The listing builds one solid part. Answer for the finished solid, in the listing's coordinates (mm). A direction names the side the tool comes from. Coordinates: 2 decimals unless noted, no trailing zeros. Write each loop counter-clockwise with the first axis right and the second up, starting at its lowest first coordinate (ties: lowest second). Pieces come first, ordered by that corner, then holes.
from build123d import *

# Parameters (mm, degrees)
SKIZZE1_R                       = 1.25
AUFSATZ_LINEAR_AUSTRAGEN1_DEPTH = 2
SKIZZE2_W                       = 150
SKIZZE2_H                       = 52
AUFSATZ_LINEAR_AUSTRAGEN2_DEPTH = 2
SKIZZE3_W                       = 30
SKIZZE3_H                       = 20
SCHNITT_LINEAR_AUSTRAGEN1_DEPTH = 2
SKIZZE5_R                       = 1.25
SCHNITT_LINEAR_AUSTRAGEN2_DEPTH = 2


with BuildPart() as part:
    # Skizze1 → Aufsatz-Linear austragen1 (new body)
    # profile 1 of 2: a face of its own
    with BuildSketch(Plane.XY):
        with BuildLine():
            Line((148, 39.858571571), (148, 12.141428429))
            ThreePointArc((148, 12.141428429), (147.219544457, 8.268445082), (145, 5))
            ThreePointArc((145, 5), (141.731554918, 2.780455543), (137.858571571, 2))
            Line((137.858571571, 2), (12.141428429, 2))
            ThreePointArc((12.141428429, 2), (8.268445082, 2.780455543), (5, 5))
            ThreePointArc((5, 5), (2.780455543, 8.268445082), (2, 12.141428429))
            Line((2, 12.141428429), (2, 39.858571571))
            ThreePointArc((2, 39.858571571), (2.780455543, 43.731554918), (5, 47))
            Line((5, 47), (5, 52))
            Line((5, 52), (145, 52))
            Line((145, 52), (145, 47))
            ThreePointArc((145, 47), (147.219544457, 43.731554918), (148, 39.858571571))
        make_face()
    # profile 2 of 2: a face of its own
    with BuildSketch(Plane.XY):
        with BuildLine():
            ThreePointArc((148, 39.858571571), (147.219544457, 43.731554918), (145, 47))
            Line((145, 47), (145, 52))
            Line((145, 52), (150, 52))
            Line((150, 52), (150, 0))
            Line((150, 0), (0, 0))
            Line((0, 0), (0, 52))
            Line((0, 52), (5, 52))
            Line((5, 52), (5, 47))
            ThreePointArc((5, 47), (2.780455543, 43.731554918), (2, 39.858571571))
            Line((2, 39.858571571), (2, 12.141428429))
            ThreePointArc((2, 12.141428429), (2.780455543, 8.268445082), (5, 5))
            ThreePointArc((5, 5), (8.268445082, 2.780455543), (12.141428429, 2))
            Line((12.141428429, 2), (137.858571571, 2))
            ThreePointArc((137.858571571, 2), (141.731554918, 2.780455543), (145, 5))
            ThreePointArc((145, 5), (147.219544457, 8.268445082), (148, 12.141428429))
            Line((148, 12.141428429), (148, 39.858571571))
        make_face()
        with Locations((2.5, 49.5)):
            Circle(SKIZZE1_R, mode=Mode.SUBTRACT)
        with Locations((2.5, 2.5)):
            Circle(SKIZZE1_R, mode=Mode.SUBTRACT)
        with Locations((147.5, 49.5)):
            Circle(SKIZZE1_R, mode=Mode.SUBTRACT)
        with Locations((147.5, 2.5)):
            Circle(SKIZZE1_R, mode=Mode.SUBTRACT)
    extrude(amount=AUFSATZ_LINEAR_AUSTRAGEN1_DEPTH)

    # Skizze2 → Aufsatz-Linear austragen2 (add)
    with BuildSketch(Plane(origin=(0, 52, 0), x_dir=(1, 0, 0), z_dir=(0, 1, 0))):
        with Locations((75, 24)):
            Rectangle(SKIZZE2_W, SKIZZE2_H)
    extrude(amount=AUFSATZ_LINEAR_AUSTRAGEN2_DEPTH)

    # Skizze3 → Schnitt-Linear austragen1 (cut)
    with BuildSketch(Plane.XZ.offset(-52)):
        with Locations((115, -40)):
            Rectangle(SKIZZE3_W, SKIZZE3_H)
    extrude(amount=-SCHNITT_LINEAR_AUSTRAGEN1_DEPTH, mode=Mode.SUBTRACT)

    # Skizze5 → Schnitt-Linear austragen2 (cut)
    with BuildSketch(Plane(origin=(0, 54, 0), x_dir=(1, 0, 0), z_dir=(0, 1, 0))):
        with Locations(Location((147.5, 47.5, 0), (0, 0, 270))):
            Circle(SKIZZE5_R)
        with Locations(Location((2.5, 47.5, 0), (0, 0, 270))):
            Circle(SKIZZE5_R)
    extrude(amount=-SCHNITT_LINEAR_AUSTRAGEN2_DEPTH, mode=Mode.SUBTRACT)


solid = part.part
1. Flat-ended cylindrical pins translate along their axes: P1, Ø2, axis at x = 147.5, y = 2.5, coming from the -Z side; P2, Ø15.5, axis at x = 108.5, y = 20.5, coming from the -Z side; P3, Ø3, axis at x = 147.5, z = -47.5, coming from the -Y side; P4, Ø1.6, axis at x = 116.5, y = 53.5, coming from the -Z side. Find the tip coordinate at first contact, or state that the pin passes through.
Results found:
P1: passes through
P2: stops at z = 0
P3: stops at y = 52
P4: stops at z = -30
2. A tool of negligible diameter and unlimited length cuts with its end or side. For faces 1 (the flat face through (74, 54, -24)), 2 (the flat face through (76, 26, 0)), from which of +Z, -Z, +X, -X, +Y, -Y can it reach the whole face along a straight path? Write none if from no direction.
Results found:
face 1: +Z, -Z, +X, -X, +Y
face 2: -Z, +X, -X, -Y
3. Section B-B on x = 74 is taken. Give the vertices of the cut face in (y, z), then the cut area to 3 significant figures.
Results found:
outline: (0, 0) - (52, 0) - (52, -50) - (54, -50) - (54, 2) - (0, 2) - close
area: 208 mm2
4. Section A-A on z = -34 is taken. Give the vertices of the cut face in (x, y).
Results found:
outline: (0, 52) - (100, 52) - (100, 54) - (0, 54) - close; (130, 52) - (150, 52) - (150, 54) - (130, 54) - close
5. Section D-D on z = -17.5 is taken. Give the vertices of the cut face in (x, y).
Results found:
outline: (0, 52) - (150, 52) - (150, 54) - (0, 54) - close
6. Find the intervals of material crossed by L1, parallel to Y at x = 147.5, z = 1.5; L2, parallel to X at y = 53, z = -47; L3, parallel to Y at x = 76.5, z = -20, in increasing order.
Results found:
L1: y = 0 to 1.25, 3.75 to 48.25, 50.75 to 54
L2: x = 0 to 1.35, 3.65 to 100, 130 to 146.35, 148.65 to 150
L3: y = 52 to 54
7. Section C-C on y = 33 is taken. Give the vertices of the cut face in (x, z), then the cut area to 3 significant figures.
Results found:
outline: (0, 0) - (150, 0) - (150, 2) - (0, 2) - close
area: 300 mm2
